```python
from build123d import *

# Parameters (mm, degrees)
BOSS_EXTRUDE2_DEPTH = 8
SKETCH2_R           = 2
CUT_EXTRUDE1_DEPTH  = 20
SKETCH3_R           = 3.5
CUT_EXTRUDE2_DEPTH  = 15


with BuildPart() as part:
    # Sketch1 → Boss-Extrude2 (new body)
    with BuildSketch(Plane.XY):
        with BuildLine():
            Line((-56.573708053, 24.587270805), (1.087717528, 24.587270805))
            Line((1.087717528, 24.587270805), (1.087717528, 22.787270805))
            ThreePointArc((1.087717528, 22.787270805), (-1.112282472, 20.587270805), (1.087717528, 18.387270805))
            Line((1.087717528, 18.387270805), (6.087717528, 18.387270805))
            Line((6.087717528, 18.387270805), (6.087717528, 4.587270805))
            Line((6.087717528, 4.587270805), (-93.912282472, 4.587270805))
            Line((-93.912282472, 4.587270805), (-93.912282472, 18.387270805))
            Line((-93.912282472, 18.387270805), (-58.912282472, 18.387270805))
            ThreePointArc((-58.912282472, 18.387270805), (-57.356647554, 19.031635886), (-56.712282472, 20.587270805))
            ThreePointArc((-56.712282472, 20.587270805), (-56.677628479, 22.588470624), (-56.573708053, 24.587270805))
        make_face()
    extrude(amount=BOSS_EXTRUDE2_DEPTH)

    # Sketch2 → Cut-Extrude1 (cut)
    with BuildSketch(Plane(origin=(0, 24.587270805, 0), x_dir=(1, 0, 0), z_dir=(0, 1, 0))):
        with Locations(Location((-8.912282472, -4, 0), (0, 0, 270))):
            Circle(SKETCH2_R)
    extrude(amount=-CUT_EXTRUDE1_DEPTH, mode=Mode.SUBTRACT)

    # Sketch3 → Cut-Extrude2 (cut)
    with BuildSketch(Plane(origin=(0, 24.587270805, 0), x_dir=(1, 0, 0), z_dir=(0, 1, 0))):
        with Locations(Location((-8.912282472, -4, 0), (0, 0, 270))):
            Circle(SKETCH3_R)
    extrude(amount=-CUT_EXTRUDE2_DEPTH, mode=Mode.SUBTRACT)


solid = part.part
```
Here's how the part is built. I have some questions about the finished solid (model axes, mm). A direction names the side the tool comes from. Give positions to 0.01 mm unless a question says otherwise; leave off trailing zeros. Loops run counter-clockwise (first coordinate to the right, second up) from the corner with the lowest first, then second, coordinate; pieces in that order, holes last. Notation, with made-up numbers: M -28,84.5 L -17,84.5 A21 ccw -17,94.5 Z; hole C 64.5,-18.5 d10. An arc over 180 degrees is marked long. Return JSON: item names as keys, results as strings.
Item 1: Please list where these lines run through material, in increasing order: line 1 (X direction, y = 6.65, z = 4); line 2 (Y direction, x = -76, z = 5.5); line 3 (Z direction, x = -11.5, y = 13.25).
A:
{"line 1": "x = -93.91 to -10.91, -6.91 to 6.09", "line 2": "y = 4.59 to 18.39", "line 3": "z = 0 to 1.64, 6.36 to 8"}
Item 2: Imagine slicing it at C-C on x = -85. List the corners of the cut face in (y, z) for me, then the cut area to 3 significant figures.
A:
{"outline": "M 4.59,0 L 18.39,0 L 18.39,8 L 4.59,8 Z", "area": "110 mm^2"}
Item 3: Imagine slicing it at B-B on y = 6.5. List the corners of the cut face in (x, z) for me.
A:
{"outline": "M -93.91,0 L 6.09,0 L 6.09,8 L -93.91,8 Z; hole C -8.91,4 d4"}
Item 4: Imagine slicing it at D-D on y = 19.5. List the corners of the cut face in (x, z) for me.
A:
{"outline": "M -57,0 L -0.82,0 L -0.82,8 L -57,8 Z; hole C -8.91,4 d7"}
Item 5: I'm going to push flat-ended pins straight in: pin 1 Ø2 at (x, z) = (-9.5, 5) entering from +Y; pin 2 Ø0.9 at (y, z) = (24, 5) entering from +X; pin 3 Ø2 at (x, z) = (-83, 6.5) entering from +Y. Where does each tip first touch, or does it pass through?
A:
{"pin 1": "stops at y = 9.59", "pin 2": "stops at x = 1.09", "pin 3": "stops at y = 18.39"}
Item 6: On a 3-axis mill with a long thin cutter (end or side, diameter ignored), from which of +Z, -Z, +X, -X, +Y, -Y can I reach the whole of each face in a straight line? I mean faces 4 (the cylindrical face through (-10.253, 17.192, 7.233)), 5 (the flat face through (-77, 18.387, 4)), 6 (the flat face through (1.088, 24, 4)). Say none if no direction works.
A:
{"face 4": "+Y", "face 5": "+Z, -Z, -X, +Y", "face 6": "+Z, -Z, +X, +Y"}
Item 7: Imagine slicing it at A-A on z = 4. List the corners of the cut face in (x, y) for me, then the cut area to 3 significant figures.
A:
{"outline": "M -93.91,4.59 L -10.91,4.59 L -10.91,9.59 L -12.41,9.59 L -12.41,24.59 L -56.57,24.59 A57.8 ccw -56.71,20.59 A2.2 cw -58.91,18.39 L -93.91,18.39 Z; M -6.91,4.59 L 6.09,4.59 L 6.09,18.39 L 1.09,18.39 A2.2 cw 1.09,22.79 L 1.09,24.59 L -5.41,24.59 L -5.41,9.59 L -6.91,9.59 Z", "area": "1,610 mm^2"}
Item 8: Thinking about a two-plate mould opening in Z: for faces 1 (the flat face through (-10, 9.587, 6)), 2 (the flat face through (6.088, 12, 4)), 3 (the flat face through (-43, 13, 0)), which applies, released by +Z, released by -Z, zero draft, split by the parting line, or undercut?
A:
{"face 1": "undercut", "face 2": "zero draft", "face 3": "released by -Z"}
